```python
from build123d import *

# Parameters (mm, degrees)
SKIZZE1_R                       = 9.5
SKIZZE1_R_2                     = 5
AUFSATZ_LINEAR_AUSTRAGEN1_DEPTH = 29
SKIZZE2_R                       = 9
SKIZZE2_R_2                     = 5.5
SCHNITT_LINEAR_AUSTRAGEN1_DEPTH = 0.5
SKIZZE3_R                       = 9
SKIZZE3_R_2                     = 5.5
SCHNITT_LINEAR_AUSTRAGEN2_DEPTH = 0.5


with BuildPart() as part:
    # Skizze1 → Aufsatz-Linear austragen1 (new body)
    with BuildSketch(Plane.XY):
        Circle(SKIZZE1_R)
        Circle(SKIZZE1_R_2, mode=Mode.SUBTRACT)
    extrude(amount=-AUFSATZ_LINEAR_AUSTRAGEN1_DEPTH)

    # Skizze2 → Schnitt-Linear austragen1 (cut)
    with BuildSketch(Plane.XY):
        Circle(SKIZZE2_R)
        Circle(SKIZZE2_R_2, mode=Mode.SUBTRACT)
    extrude(amount=-SCHNITT_LINEAR_AUSTRAGEN1_DEPTH, mode=Mode.SUBTRACT)

    # Skizze3 → Schnitt-Linear austragen2 (cut)
    with BuildSketch(Plane(origin=(0, 0, -29), x_dir=(-1, 0, 0), z_dir=(0, 0, -1))):
        Circle(SKIZZE3_R)
        Circle(SKIZZE3_R_2, mode=Mode.SUBTRACT)
    extrude(amount=-SCHNITT_LINEAR_AUSTRAGEN2_DEPTH, mode=Mode.SUBTRACT)


solid = part.part
```
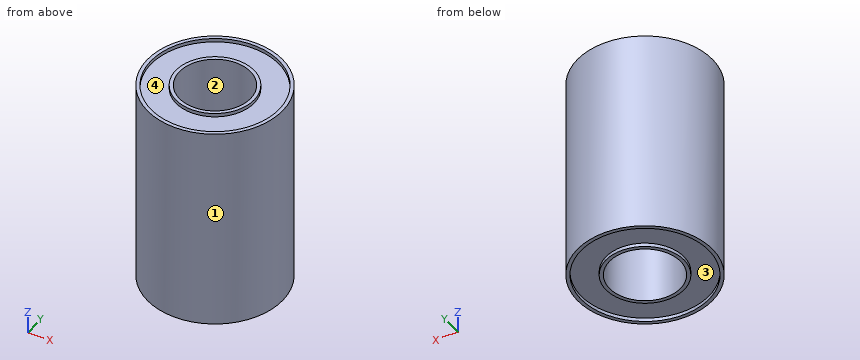
Model file for the job. Use its own axes, mm. Face numbers are marked on the shaded views. A direction names the side the tool comes from. Coordinates: 2 decimals unless noted, no trailing zeros. Loops run counter-clockwise (first coordinate to the right, second up) from the corner with the lowest first, then second, coordinate; pieces in that order, holes last. Notation, with made-up numbers: (40.25, 51.5) - (78.25, 51.5) arc R18 ccw to (78.25, 81.5) - close; hole circle Ø5 at (81, 82). An arc over 180 degrees is marked (long way). Answer as a JSON object with one key per item and string values. Group by question number.
(1) Flat gauge pins, fed straight in: pin 1 (4 mm diameter, centred on y = -2.5, z = -17, fed in from +X); pin 2 (4 mm diameter, centred on x = -5.5, z = -5.5, fed in from +Y); pin 3 (1.5 mm diameter, centred on x = -4, z = -21, fed in from +Y). Where does each tip first touch, or does it go through?
(2) Cut at C-C (z = -11). Give the cut face in (x, y).
(3) Tool access for the marked faces 3 and 4: list every direction of +Z, -Z, +X, -X, +Y, -Y with a clear straight run to the whole face (end or side of a thin tool).
(4) Probe line 1 along Y through (x, z) = (0, -28.7); line 2 along Y through (x, z) = (0, -9.75); line 3 along Z through (x, y) = (6.5, -4.5). List the from-to ranges inside material, lowest first.
(5) Cut at D-D (x = 8.25). Give the cut face in (y, z), then the cut area to 3 significant figures.
(6) Cut at A-A (x = 0). Give the cut face in (y, z), then the cut area to 3 significant figures.
(7) Two-plate mould, pull along X, no slides. Class the marked faces 1 and 2: released by +X, released by -X, zero draft, split by the parting line, or undercut.
Geometry says:
{
 "1": {"pin 1": "stops at x = 9.49", "pin 2": "stops at y = 8.83", "pin 3": "stops at y = 8.93"},
 "2": {"outline": "circle Ø19 at (0, 0); hole circle Ø10 at (0, 0)"},
 "3": {"face 3": "-Z", "face 4": "+Z"},
 "4": {"line 1": "y = -9.5 to -9, -5.5 to -5, 5 to 5.5, 9 to 9.5", "line 2": "y = -9.5 to -5, 5 to 9.5", "line 3": "z = -28.5 to -0.5"},
 "5": {"outline": "(-4.71, -29) - (-3.6, -29) - (-3.6, -28.5) - (3.6, -28.5) - (3.6, -29) - (4.71, -29) - (4.71, 0) - (3.6, 0) - (3.6, -0.5) - (-3.6, -0.5) - (-3.6, 0) - (-4.71, 0) - close", "area": "266 mm^2"},
 "6": {"outline": "(-9.5, -29) - (-9, -29) - (-9, -28.5) - (-5.5, -28.5) - (-5.5, -29) - (-5, -29) - (-5, 0) - (-5.5, 0) - (-5.5, -0.5) - (-9, -0.5) - (-9, 0) - (-9.5, 0) - close; (5, -29) - (5.5, -29) - (5.5, -28.5) - (9, -28.5) - (9, -29) - (9.5, -29) - (9.5, 0) - (9, 0) - (9, -0.5) - (5.5, -0.5) - (5.5, 0) - (5, 0) - close", "area": "254 mm^2"},
 "7": {"face 1": "split by the parting line", "face 2": "undercut"}
}
